Verification items for the finished model (mm, model axes). Face numbers are marked on the shaded views. Coordinates: 2 decimals unless noted, no trailing zeros. Write each loop counter-clockwise with the first axis right and the second up, starting at its lowest first coordinate (ties: lowest second). Pieces come first, ordered by that corner, then holes. Notation, with made-up numbers: (18.5, 42.25) -> (69.5, 42.25) arc R9 ccw to (69.5, 59.25) -> close; hole circle Ø10 at (20.25, 1.25). An arc over 180 degrees is marked (long way). Use CSV: the item, a comma, the result in double quotes.
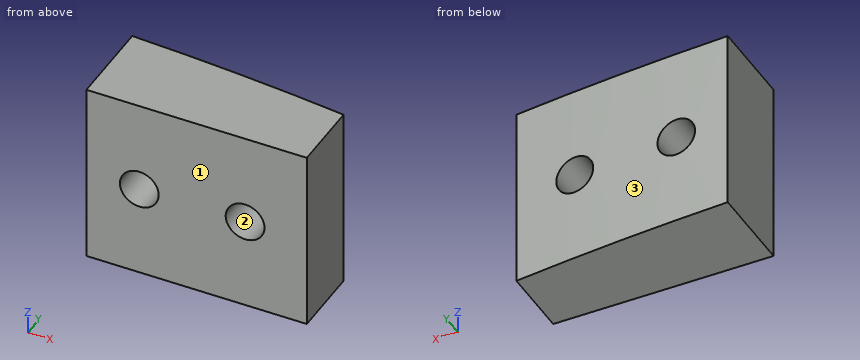
```python
from build123d import *

# Parameters (mm, degrees)
BOSS_EXTRU_1_DEPTH = 15.75
D_GAGEMENT_M61_D   = 6.6


with BuildPart() as part:
    # Esquisse1 → Boss.-Extru.1 (new body, symmetric)
    with BuildSketch(Plane.XY):
        with BuildLine():
            Line((0, 0), (37.5, 0))
            Line((37.5, 0), (37.5, 12.2))
            ThreePointArc((37.5, 12.2), (18.778224846, 14.052810579), (0, 15.2))
            Line((0, 15.2), (0, 0))
        make_face()
    extrude(amount=BOSS_EXTRU_1_DEPTH, both=True)

    # Dégagement M61 (through all)
    with Locations(Plane(origin=(0, 0, 0), x_dir=(-1, 0, 0), z_dir=(0, -1, 0))):
        with Locations((-9, 0), (-27, 0)):
            Hole(D_GAGEMENT_M61_D / 2)


solid = part.part
```
1) Gauge pin test, flat ends, axial feed: pin 1 (7.5 mm diameter, centred on x = 27, z = 0, fed in from +Y); pin 2 (8 mm diameter, centred on x = 18, z = -11.5, fed in from +Y); pin 3 (5 mm diameter, centred on x = 32, z = 3, fed in from +Y); pin 4 (12 mm diameter, centred on x = 33, z = 5, fed in from -Y). Record the tip position at first contact, or that the pin passes through.
Return value:
pin 1,"y = 13.67"
pin 2,"y = 14.41"
pin 3,"y = 13.08"
pin 4,"y = 0"
2) Cross-section at B-B (y = 7). Record the boundary of the cut face in (x, z).
Return value:
outline,"(0, -15.75) -> (37.5, -15.75) -> (37.5, 15.75) -> (0, 15.75) -> close; hole circle Ø6.6 at (9, 0); hole circle Ø6.6 at (27, 0)"
3) Cross-section at D-D (x = 9). Record the boundary of the cut face in (y, z), plus the area to 3 significant figures.
Return value:
outline,"(0, -15.75) -> (14.74, -15.75) -> (14.74, -3.3) -> (0, -3.3) -> close; (0, 3.3) -> (14.74, 3.3) -> (14.74, 15.75) -> (0, 15.75) -> close"
area,"367 mm2"
4) Cross-section at C-C (z = 0). Record the boundary of the cut face in (x, y), plus the area to 3 significant figures.
Return value:
outline,"(0, 0) -> (5.7, 0) -> (5.7, 14.93) arc R500 ccw to (0, 15.2) -> close; (12.3, 0) -> (23.7, 0) -> (23.7, 13.63) arc R500 ccw to (12.3, 14.53) -> close; (30.3, 0) -> (37.5, 0) -> (37.5, 12.2) arc R500 ccw to (30.3, 13) -> close"
area,"337 mm2"
5) Scan lines: L1, parallel to Z at x = 9, y = 11.5; L2, parallel to Z at x = 29, y = 11; L3, parallel to Y at x = 2, z = -6. Record each from-to range of solid material in increasing order.
Return value:
L1,"-15.75 to -3.3, 3.3 to 15.75"
L2,"-15.75 to -2.62, 2.62 to 15.75"
L3,"0 to 15.11"
6) Cross-section at A-A (x = 27). Record the boundary of the cut face in (y, z), plus the area to 3 significant figures.
Return value:
outline,"(0, -15.75) -> (13.33, -15.75) -> (13.33, -3.3) -> (0, -3.3) -> close; (0, 3.3) -> (13.33, 3.3) -> (13.33, 15.75) -> (0, 15.75) -> close"
area,"332 mm2"
7) Mould release check, pull along X, two halves, no side actions. Record for the marked faces 1, 2 and 3: released by +X, released by -X, zero draft, split by the parting line, or undercut.
Return value:
face 1,"zero draft"
face 2,"undercut"
face 3,"released by +X"
